from build123d import *

# Parameters (mm, degrees)
F0_R     = 1.5
F0_R_2   = 2.6
F1_DEPTH = 1.6


with BuildPart() as f1:
    # F0 (on Top) → F1 (new body)
    with BuildSketch(Plane.XY):
        Polygon((9.5, 50), (-9.5, 50), (-9.5, 9.5), (-50, 9.5), (-50, -9.5), (-9.5, -9.5), (-9.5, -50), (9.5, -50), (9.5, -9.5), (50, -9.5), (50, 9.5), (9.5, 9.5), align=None)
        with Locations((-6, -6)):
            Circle(F0_R, mode=Mode.SUBTRACT)
        with Locations((0, -45)):
            Circle(F0_R_2, mode=Mode.SUBTRACT)
        with Locations((6, -6)):
            Circle(F0_R, mode=Mode.SUBTRACT)
        with Locations((-45, 0)):
            Circle(F0_R_2, mode=Mode.SUBTRACT)
        with Locations((-6, 6)):
            Circle(F0_R, mode=Mode.SUBTRACT)
        with Locations((6, 6)):
            Circle(F0_R, mode=Mode.SUBTRACT)
        with Locations((45, 0)):
            Circle(F0_R_2, mode=Mode.SUBTRACT)
        with Locations((0, 45)):
            Circle(F0_R_2, mode=Mode.SUBTRACT)
    extrude(amount=F1_DEPTH)


solid = f1.part
The listing builds one solid part. Answer for the finished solid, in the listing's coordinates (mm). Round coordinates to 2 decimals unless told otherwise and drop trailing zeros. Write each loop counter-clockwise with the first axis right and the second up, starting at its lowest first coordinate (ties: lowest second). Pieces come first, ordered by that corner, then holes. Notation, with made-up numbers: M -40,77 L -23,77 A23 ccw -23,92 Z; hole C 69,56 d5. An arc over 180 degrees is marked long. Write each question's results on one line, items separated by ' | '. Start each with the question number.
(1) Each of these flat-tipped pins is pushed along its axis until it touches: P1, Ø0.5, axis at y = -25.5, z = 0.5, coming from the +X side; P2, Ø2.5, axis at x = -6, y = 6, coming from the +Z side; P3, Ø0.8, axis at y = -23.5, z = 1, coming from the -X side. Where does it stop, or does it pass through?
(2) Determine the mould class of faces 1 (the flat face through (0, 4, 0)), 2 (the cylindrical face through (-0.56, 42.46, 0.79)), 3 (the cylindrical face through (-0.56, -47.54, 0.79)) for opening direction X: +X half, -X half, draft (parallel to the pull), parting line (faces both ways), or undercut.
(3) Find the intervals of material crossed by line 1 (Y direction, x = -6, z = 1.1); line 2 (Y direction, x = -45, z = 0.5); line 3 (Y direction, x = -33, z = 1.55), in increasing order.
(4) The part is cut by section A-A, the plane y = -6. Write down the section's boundary in (x, z), and give its area (3 significant figures).
(5) The part is cut by section B-B, the plane x = 45. Write down the section's boundary in (y, z).
(6) The part is cut by section D-D, the plane x = 0. Write down the section's boundary in (y, z), and give its area (3 significant figures).
Worked answers:
1) P1: stops at x = 9.5 | P2: passes through | P3: stops at x = -9.5
2) face 1: draft | face 2: undercut | face 3: undercut
3) line 1: y = -50 to -7.5, -4.5 to 4.5, 7.5 to 50 | line 2: y = -9.5 to -2.6, 2.6 to 9.5 | line 3: y = -9.5 to 9.5
4) outline: M -50,0 L -7.5,0 L -7.5,1.6 L -50,1.6 Z; M -4.5,0 L 4.5,0 L 4.5,1.6 L -4.5,1.6 Z; M 7.5,0 L 50,0 L 50,1.6 L 7.5,1.6 Z | area: 150 mm²
5) outline: M -9.5,0 L -2.6,0 L -2.6,1.6 L -9.5,1.6 Z; M 2.6,0 L 9.5,0 L 9.5,1.6 L 2.6,1.6 Z
6) outline: M -50,0 L -47.6,0 L -47.6,1.6 L -50,1.6 Z; M -42.4,0 L 42.4,0 L 42.4,1.6 L -42.4,1.6 Z; M 47.6,0 L 50,0 L 50,1.6 L 47.6,1.6 Z | area: 143 mm²
